from build123d import *

# Parameters (mm, degrees)
F0_W     = 68
F0_H     = 78
F1_DEPTH = 30
F2_T     = -3
F3_W     = 80
F3_H     = 30
F4_DEPTH = 6
F5_SIZE2 = 1
F5_SIZE  = 3
F8_R     = 3


with BuildPart() as f1:
    # F0 (on Top) → F1 (new body)
    with BuildSketch(Plane.XY):
        with Locations((0, 39)):
            Rectangle(F0_W, F0_H)
    extrude(amount=F1_DEPTH)

    # F2
    f2_openings = [f1.faces().sort_by_distance(p)[0] for p in [
        (0, 39, 30),
        (0, 0, 15),
    ]]
    offset(amount=F2_T, openings=f2_openings)

    # F3 (on Front) → F4 (join)
    with BuildSketch(Plane.XZ):
        with Locations((0, 15)):
            Rectangle(F3_W, F3_H)
    extrude(amount=F4_DEPTH)

    # F5
    f5_edges = [f1.edges().sort_by_distance(p)[0] for p in [
        (0, -6, 30),
        (-40, -6, 15),
        (0, -6, 0),
        (40, -6, 15),
    ]]
    f5_side = f1.faces().sort_by_distance((0, -6, 15))[0]
    chamfer(f5_edges, length=F5_SIZE, length2=F5_SIZE2, reference=f5_side)

    # F6 (on Right) → F7 (revolve)
    with BuildSketch(Plane.YZ):
        with BuildLine():
            ThreePointArc((-20.9666295471, 25), (-23.2249721603, 20.2249721603), (-24, 15))
            Line((-24, 15), (-6, 15))
            Line((-6, 15), (-6, 22.5))
            Line((-6, 22.5), (-20.9666295471, 25))
        make_face()
    revolve(axis=Axis((0, -21.969004482, 15), (0, -1, 0)))

    # F8
    f8_edges = [f1.edges().sort_by_distance(p)[0] for p in [
        (0, -20.96663, 5),
    ]]
    fillet(f8_edges, radius=F8_R)


solid = f1.part
The listing builds one solid part. Answer for the finished solid, in the listing's coordinates (mm). A direction names the side the tool comes from. Give positions to 0.01 mm unless a question says otherwise; leave off trailing zeros. Write each loop counter-clockwise with the first axis right and the second up, starting at its lowest first coordinate (ties: lowest second). Pieces come first, ordered by that corner, then holes.
1) Given P1, Ø2, axis at y = 60, z = 11, coming from the -X side; P2, Ø5, axis at x = -38, z = 11.5, coming from the +Y side; P3, Ø1.5, axis at x = -10.5, z = 12.5, coming from the -Y side; P4, Ø12, axis at x = -2, z = 11.5, coming from the -Y side, each flat-ended and moving along its own axis, determine where each tip first touches the part or whether it passes through.
2) For a pull along X with two mould halves and no side action, classify faces 6 (the face through (31, 37, 16)), 7 (the face through (40, -2, 15)), 8 (the face through (-0.2, -0.2, 30)) as pulls with the +X half, pulls with the -X half, needs draft (parallel to the pull), parting line crosses it, or undercut.
3) Find the intervals of material crossed by L1, parallel to Y at x = 20, z = 27; L2, parallel to X at y = 16, z = 7.5; L3, parallel to Y at x = -33, z = 15.5, in increasing order.
4) A tool of negligible diameter and unlimited length cuts with its end or side. For faces 1 (the face through (-2.51, -11.12, 22.97)), 2 (the face through (0, 0, 17)), 3 (the face through (-0.6, -5.5, 1.5)), 4 (the face through (37, 0, 15)), 5 (the face through (-37, 0, 15)), from which of +Z, -Z, +X, -X, +Y, -Y can it reach the whole face along a straight path? Write none if from no direction.
5) Section A-A (y = 35) is taken. Write down the section's boundary in (x, z), and give its area (3 significant figures).
Response:
1. P1: stops at x = -34
1. P2: stops at y = 0
1. P3: stops at y = -6
1. P4: stops at y = -24
2. face 6: undercut
2. face 7: pulls with the +X half
2. face 8: needs draft
3. L1: y = -6 to 0, 75 to 78
3. L2: x = -34 to -31, 31 to 34
3. L3: y = -6 to 78
4. face 1: none
4. face 2: +Z
4. face 3: -Z, +X, -X, -Y
4. face 4: +Z, -Z, +X, +Y
4. face 5: +Z, -Z, -X, +Y
5. outline: (-34, 0) - (34, 0) - (34, 30) - (31, 30) - (31, 3) - (-31, 3) - (-31, 30) - (-34, 30) - close
5. area: 366 mm2
